from build123d import *

# Parameters (mm, degrees)
SKETCH1_W           = 40
SKETCH1_H           = 19
SKETCH1_R           = 2.75
BOSS_EXTRUDE1_DEPTH = 4
SKETCH2_R           = 7.1705
BOSS_EXTRUDE2_DEPTH = 26
SKETCH3_R           = 5.5
BOSS_EXTRUDE3_DEPTH = 22
SKETCH4_R           = 7.1705
BOSS_EXTRUDE4_DEPTH = 5


with BuildPart() as part:
    # Sketch1 → Boss-Extrude1 (new body)
    with BuildSketch(Plane.XY):
        Rectangle(SKETCH1_W, SKETCH1_H)
        with Locations((12, 0)):
            Circle(SKETCH1_R, mode=Mode.SUBTRACT)
        with Locations((-12, 0)):
            Circle(SKETCH1_R, mode=Mode.SUBTRACT)
    extrude(amount=-BOSS_EXTRUDE1_DEPTH)

    # Sketch2 → Boss-Extrude2 (add)
    with BuildSketch(Plane.XY):
        Circle(SKETCH2_R)
    extrude(amount=BOSS_EXTRUDE2_DEPTH)

    # Sketch3 → Boss-Extrude3 (add)
    with BuildSketch(Plane.XY.offset(26)):
        Circle(SKETCH3_R)
    extrude(amount=BOSS_EXTRUDE3_DEPTH)

    # Sketch4 → Boss-Extrude4 (add)
    with BuildSketch(Plane.XY.offset(48)):
        Circle(SKETCH4_R)
    extrude(amount=BOSS_EXTRUDE4_DEPTH)


solid = part.part
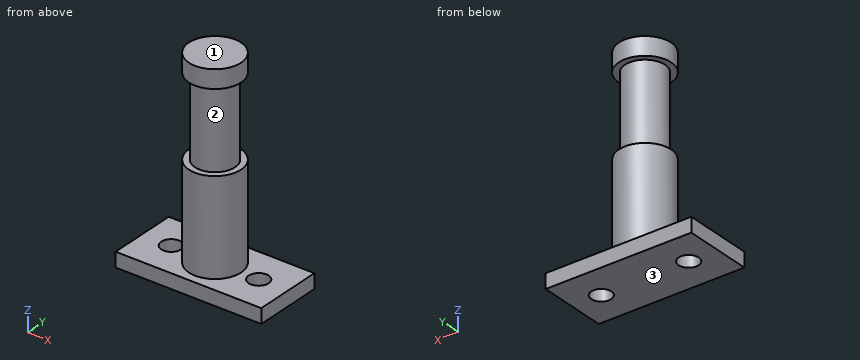
CAD build for the part. Positions are in the model's coordinates, mm. Face numbers are marked on the shaded views. Give positions to 0.01 mm unless a question says otherwise; leave off trailing zeros. Order: outer loops, then holes, each group sorted by start corner. A loop starts at its lowest first (then second) coordinate and runs counter-clockwise, first axis right, second up. Notation, with made-up numbers: (82, 49) - (135, 49) arc R34 ccw to (135, 85) - close; hole circle Ø1 at (-28, 32.5). An arc over 180 degrees is marked (long way). Answer in a Markdown table with one row per item.
1. Saw through at D-D, the plane x = 0. Give the cut face in (y, z).
Data:
| item | result |
|---|---|
| outline | (-9.5, -4) - (9.5, -4) - (9.5, 0) - (7.17, 0) - (7.17, 26) - (5.5, 26) - (5.5, 48) - (7.17, 48) - (7.17, 53) - (-7.17, 53) - (-7.17, 48) - (-5.5, 48) - (-5.5, 26) - (-7.17, 26) - (-7.17, 0) - (-9.5, 0) - close |
2. Saw through at C-C, the plane z = 21. Give the cut face in (x, y), plus the area to 3 significant figures.
Data:
| item | result |
|---|---|
| outline | circle Ø14.34 at (0, 0) |
| area | 162 mm² |
3. Saw through at B-B, the plane y = 0. Give the cut face in (x, z), plus the area to 3 significant figures.
Data:
| item | result |
|---|---|
| outline | (-20, -4) - (-14.75, -4) - (-14.75, 0) - (-20, 0) - close; (-9.25, -4) - (9.25, -4) - (9.25, 0) - (7.17, 0) - (7.17, 26) - (5.5, 26) - (5.5, 48) - (7.17, 48) - (7.17, 53) - (-7.17, 53) - (-7.17, 48) - (-5.5, 48) - (-5.5, 26) - (-7.17, 26) - (-7.17, 0) - (-9.25, 0) - close; (14.75, -4) - (20, -4) - (20, 0) - (14.75, 0) - close |
| area | 803 mm² |
4. Pull direction Z, two halves, no side cores. Call the marked faces 1, 2 and 3: pulls with the +Z half, pulls with the -Z half, needs draft (parallel to the pull), parting line crosses it, or undercut.
Data:
| item | result |
|---|---|
| face 1 | pulls with the +Z half |
| face 2 | undercut |
| face 3 | pulls with the -Z half |
5. Saw through at A-A, the plane x = -12. Give the cut face in (y, z).
Data:
| item | result |
|---|---|
| outline | (-9.5, -4) - (-2.75, -4) - (-2.75, 0) - (-9.5, 0) - close; (2.75, -4) - (9.5, -4) - (9.5, 0) - (2.75, 0) - close |
6. Flat gauge pins, fed straight in: pin 1 (10 mm diameter, centred on x = 8, z = 9.5, fed in from -Y); pin 2 (1 mm diameter, centred on y = 5, z = 26, fed in from +X); pin 3 (1.5 mm diameter, centred on x = -11.5, y = 0, fed in from -Z); pin 4 (6.5 mm diameter, centred on x = -12, y = 0, fed in from +Z). Where does each tip first touch, or does it go through?
Data:
| item | result |
|---|---|
| pin 1 | stops at y = -6.51 |
| pin 2 | stops at x = 5.58 |
| pin 3 | passes through |
| pin 4 | stops at z = 0 |
7. Probe probe 1 along Y at (x, z) = (12, -1); probe 2 along Z at (x, y) = (4, -4.25); probe 3 along Z at (x, y) = (12.5, 7.5). List the from-to ranges inside material, lowest first. Write a range as [from, to].
Data:
| item | result |
|---|---|
| probe 1 | y = [-9.5, -2.75], [2.75, 9.5] |
| probe 2 | z = [-4, 26], [48, 53] |
| probe 3 | z = [-4, 0] |
